from build123d import *

# Parameters (mm, degrees)
BOSS_EXTRUDE1_DEPTH = 2.5
FILLET1_R           = 3
FILLET2_R           = 1


with BuildPart() as part:
    # Sketch1 → Boss-Extrude1 (new, symmetric)
    with BuildSketch(Plane.XY):
        with BuildLine():
            Line((17.636964024, 2), (25.636964024, 2))
            ThreePointArc((25.636964024, 2), (27.636964024, 0), (25.636964024, -2))
            Line((25.636964024, -2), (21.636964024, -7.712592027))
            Line((21.636964024, -7.712592027), (25.636964024, -18.702501705))
            Line((25.636964024, -18.702501705), (28.136964024, -21.702501705))
            Line((28.136964024, -21.702501705), (30.636964024, -18.702501705))
            Line((30.636964024, -18.702501705), (30.636964024, 0))
            ThreePointArc((30.636964024, 0), (29.636964024, 1), (30.636964024, 2))
            Line((30.636964024, 2), (30.636964024, 5))
            Line((30.636964024, 5), (9.886964024, 25.75))
            Line((9.886964024, 25.75), (-9.886964024, 25.75))
            Line((-9.886964024, 25.75), (-30.636964024, 5))
            Line((-30.636964024, 5), (-30.636964024, 2))
            ThreePointArc((-30.636964024, 2), (-29.636964024, 1), (-30.636964024, 0))
            Line((-30.636964024, 0), (-30.636964024, -18.702501705))
            Line((-30.636964024, -18.702501705), (-28.136964024, -21.702501705))
            Line((-28.136964024, -21.702501705), (-25.636964024, -18.702501705))
            Line((-25.636964024, -18.702501705), (-21.636964024, -7.712592027))
            Line((-21.636964024, -7.712592027), (-25.636964024, -2))
            ThreePointArc((-25.636964024, -2), (-27.636964024, 0), (-25.636964024, 2))
            Line((-25.636964024, 2), (-17.636964024, 2))
            ThreePointArc((-17.636964024, 2), (0, 17.75), (17.636964024, 2))
        make_face()
    extrude(amount=BOSS_EXTRUDE1_DEPTH, both=True)

    # Fillet1
    fillet1_edges = [part.edges().sort_by_distance(p)[0] for p in [
        (-25.636964024, -18.702501705, 0),
        (-30.636964024, 5, 0),
        (-9.886964024, 25.75, 0),
        (9.886964024, 25.75, 0),
        (30.636964024, 5, 0),
        (25.636964024, -18.702501705, 0),
        (17.636964024, 2, 0),
        (-17.636964024, 2, 0),
    ]]
    fillet(fillet1_edges, radius=FILLET1_R)

    # Fillet2
    fillet2_edges = [part.edges().sort_by_distance(p)[0] for p in [
        (-21.636964024, -7.712592027, 0),
        (21.636964024, -7.712592027, 0),
    ]]
    fillet(fillet2_edges, radius=FILLET2_R)


solid = part.part
Geometry: final body of the model. Coordinates: model frame, mm. A direction names the side the tool comes from. Round coordinates to 2 decimals unless told otherwise and drop trailing zeros. Write each loop counter-clockwise with the first axis right and the second up, starting at its lowest first coordinate (ties: lowest second). Pieces come first, ordered by that corner, then holes. Notation, with made-up numbers: M -17,5.25 L 36,5.25 A18 cw 36,11.25 Z; hole C 51.25,-35 d5. An arc over 180 degrees is marked long. Write item = value, one per line.
Item 1: Pin query (flat end, axial travel): P1, Ø1.5, axis at y = 15, z = 1, coming from the +X side; P2, Ø1.5, axis at x = -1, z = -0.5, coming from the -Y side. Return the tip coordinate at first contact, or that it passes through.
Findings:
P1 = 21.39
P2 = 17.66
Item 2: Pull-direction query (Y, two-part tool) for faces 1 (the face through (-29.637, 1.022, 0.035)), 2 (the face through (9.777, 25.528, 0.035)), 3 (the face through (30.637, 3, 0)), 4 (the face through (18.31, 2.62, -0.04)); classes: pulls with the +Y half, pulls with the -Y half, needs draft (parallel to the pull), parting line crosses it, or undercut.
Findings:
face_1 = undercut
face_2 = pulls with the +Y half
face_3 = needs draft
face_4 = pulls with the -Y half
Item 3: Section query C-C on y = 1. Return loops of the section in (x, z).
Findings:
outline = M -29.64,-2.5 L -27.37,-2.5 L -27.37,2.5 L -29.64,2.5 Z; M 27.37,-2.5 L 29.64,-2.5 L 29.64,2.5 L 27.37,2.5 Z
Item 4: Section query D-D on x = -5.5. Return loops of the section in (y, z).
Findings:
outline = M 16.88,-2.5 L 25.75,-2.5 L 25.75,2.5 L 16.88,2.5 Z
Item 5: Material intervals for line 1 along X through (y, z) = (-17, -1.4); line 2 along X through (y, z) = (4, 0.1); line 3 along Y through (x, z) = (-21.5, 0.75), sorted ascending. Write a range as [from, to].
Findings:
line_1 = [-30.64, -25.02], [25.02, 30.64]
line_2 = [-30.63, -17.31], [17.31, 30.63]
line_3 = [2, 14.14]
Item 6: Section query A-A on y = 7.5. Return loops of the section in (x, z).
Findings:
outline = M -28.14,-2.5 L -16.09,-2.5 L -16.09,2.5 L -28.14,2.5 Z; M 16.09,-2.5 L 28.14,-2.5 L 28.14,2.5 L 16.09,2.5 Z
Item 7: Access query for faces 5 (the face through (23.81, -4.61, 0.04)), 6 (the face through (-27.07, -20.42, 0.04)), 7 (the face through (29.637, 0.978, 0.035)). Directions: +Z, -Z, +X, -X, +Y, -Y. A direction counts if a zero-diameter tool reaches every point of the face in a straight line with its end or side. Return the directions, or none.
Findings:
face_5 = +Z, -Z
face_6 = +Z, -Z, -Y
face_7 = +Z, -Z, +X
